Verification items for the finished model (mm, model axes). Give positions to 0.01 mm unless a question says otherwise; leave off trailing zeros. Order: outer loops, then holes, each group sorted by start corner. A loop starts at its lowest first (then second) coordinate and runs counter-clockwise, first axis right, second up.
(1) Scan lines: L1, parallel to Y at x = -24.5, z = 1.45; L2, parallel to Y at x = 50, z = 1.7; L3, parallel to Y at x = 25, z = 2.65. Record each from-to range of solid material in increasing order.
(2) Sectioned sample at A-A on x = 24.5. Record the cut outline in (y, z).
(3) Gauge pin test, flat end, axial feed: pin 1 (1.8 mm diameter, centred on x = 24.5, y = 29, fed in from +Z). Record the tip position at first contact, or that the pin passes through.
(4) Sectioned sample at C-C on x = 50. Record the cut outline in (y, z).
(5) Sectioned sample at B-B on y = -29. Record the cut outline in (x, z).
```python
from build123d import *

# Parameters (mm, degrees)
SKETCH_1_R      = 1.5
SKETCH_1_R_2    = 2
EXTRUDE_1_DEPTH = 3


with BuildPart() as part:
    # 草圖1 → 填料-伸長1 (new body)
    with BuildSketch(Plane.XY):
        with BuildLine():
            Line((-55, 39), (55, 39))
            ThreePointArc((55, 39), (58.535533906, 37.535533906), (60, 34))
            Line((60, 34), (60, -34))
            ThreePointArc((60, -34), (58.535533906, -37.535533906), (55, -39))
            Line((55, -39), (-55, -39))
            ThreePointArc((-55, -39), (-58.535533906, -37.535533906), (-60, -34))
            Line((-60, -34), (-60, 34))
            ThreePointArc((-60, 34), (-58.535533906, 37.535533906), (-55, 39))
        make_face()
        with Locations((-24.5, 29)):
            Circle(SKETCH_1_R, mode=Mode.SUBTRACT)
        with Locations((24.5, 29)):
            Circle(SKETCH_1_R, mode=Mode.SUBTRACT)
        with Locations((-24.5, -29)):
            Circle(SKETCH_1_R, mode=Mode.SUBTRACT)
        with Locations((24.5, -29)):
            Circle(SKETCH_1_R, mode=Mode.SUBTRACT)
        with Locations((50, 4)):
            Circle(SKETCH_1_R_2, mode=Mode.SUBTRACT)
        with Locations(Location((-50, 4, 0), (0, 0, 180))):
            Circle(SKETCH_1_R_2, mode=Mode.SUBTRACT)
    extrude(amount=EXTRUDE_1_DEPTH)


solid = part.part
```
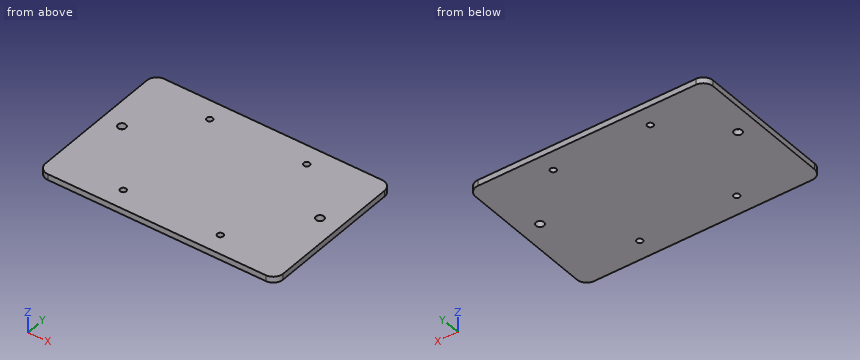
Ans:
1. L1: y = -39 to -30.5, -27.5 to 27.5, 30.5 to 39
1. L2: y = -39 to 2, 6 to 39
1. L3: y = -39 to -30.41, -27.59 to 27.59, 30.41 to 39
2. outline: (-39, 0) - (-30.5, 0) - (-30.5, 3) - (-39, 3) - close; (-27.5, 0) - (27.5, 0) - (27.5, 3) - (-27.5, 3) - close; (30.5, 0) - (39, 0) - (39, 3) - (30.5, 3) - close
3. pin 1: passes through
4. outline: (-39, 0) - (2, 0) - (2, 3) - (-39, 3) - close; (6, 0) - (39, 0) - (39, 3) - (6, 3) - close
5. outline: (-60, 0) - (-26, 0) - (-26, 3) - (-60, 3) - close; (-23, 0) - (23, 0) - (23, 3) - (-23, 3) - close; (26, 0) - (60, 0) - (60, 3) - (26, 3) - close
